Check sheet for the modelled part. Datum: model origin and axes. Units: mm. A direction names the side the tool comes from. Give positions to 0.01 mm unless a question says otherwise; leave off trailing zeros. Order: outer loops, then holes, each group sorted by start corner. A loop starts at its lowest first (then second) coordinate and runs counter-clockwise, first axis right, second up.
Autodesk Inventor part; units mm, degrees
ref_plane "YZ Plane" through (0, 0, 0) normal (1, 0, 0) x (0, 1, 0)
ref_plane "XZ Plane" through (0, 0, 0) normal (0, 1, 0) x (-1, 0, 0)
ref_plane "XY Plane" through (0, 0, 0) normal (0, 0, 1) x (1, 0, 0)
sketch "Sketch1" plane through (0, 0, 0) normal (1, 0, 0) x (0, 1, 0)
  line L0 (150, 0) -> (150, -150)
  line L1 (0, -150) -> (0, 0)
  line L2 (130, -42) -> (90, -42)
  line L3 (90, -42) -> (90, -138)
  line L4 (90, -138) -> (130, -138)
  line L5 (130, -138) -> (130, -42)
  line L6 (130, -42) -> (90, -138) construction
  line L7 (90, -42) -> (130, -138) construction
  line L8 (75, -77) -> (17, -77)
  line L9 (17, -77) -> (17, -138)
  line L10 (17, -138) -> (75, -138)
  line L11 (75, -138) -> (75, -77)
  line L12 (75, -77) -> (17, -138) construction
  line L13 (17, -77) -> (75, -138) construction
  line L14 (25, -30) -> (25, -60) construction
  line L15 (35, -30) -> (35, -60)
  line L16 (15, -60) -> (15, -30)
  arc A0 (35, -30) -> (15, -30) centre (25, -30) ccw
  arc A1 (15, -60) -> (35, -60) centre (25, -60) ccw
  line L17 (124, 0) -> (124, 10)
  line L18 (124, 10) -> (99, 10)
  line L19 (99, 10) -> (99, 0)
  line L20 (51, 0) -> (51, 10)
  line L21 (51, 10) -> (26, 10)
  line L22 (26, 10) -> (26, 0)
  line L23 (150, -75) -> (168, -75)
  line L24 (124, 0) -> (150, 0)
  line L25 (0, 0) -> (26, 0)
  line L26 (51, 0) -> (99, 0)
  line L27 (124, -150) -> (124, -160)
  line L28 (124, -160) -> (99, -160)
  line L29 (99, -160) -> (99, -150)
  line L30 (51, -150) -> (51, -160)
  line L31 (51, -160) -> (26, -160)
  line L32 (26, -160) -> (26, -150)
  line L33 (150, -150) -> (124, -150)
  line L34 (99, -150) -> (51, -150)
  line L35 (26, -150) -> (0, -150)
  point P0 (110, -90)
  point P1 (46, -107.5)
  point P2 (25, -45)
  dimension "d0" = 150
  dimension "d1" = 150
  dimension "d2" = 90
  dimension "d3" = 110
  dimension "d4" = 40
  dimension "d5" = 96
  dimension "d6" = 58
  dimension "d7" = 61
  dimension "d8" = 46
  dimension "d9" = 96
  dimension "d10" = 25
  dimension "d11" = 30
  dimension "d12" = 30
  dimension "d13" = 10
  dimension "d16" = 25
  dimension "d17" = 10
  dimension "d18" = 26
  dimension "d19" = 10
  dimension "d20" = 25
  dimension "d21" = 26
  dimension "d24" = 33
  dimension "d25" = 75
  dimension "d26" = 18
extrude "Extrusion1" add sketch "Sketch1" along normal blind 3
properties part number "front_part"
(1) Release check for a two-part mould opening along Z. For faces 1 (the face through (1, 25, -70)), 2 (the face through (0, 74, -74)) record: released by +Z, released by -Z, zero draft, split by the parting line, or undercut.
Response values:
face 1: undercut
face 2: zero draft
(2) Cross-section at C-C on x = 0.95. Count the separate pieces of the cut face and the enclosed holes in it, then the cut area to 3 significant figures.
Response values:
separate pieces: 1
enclosed holes: 3
area: 15,200 mm2
(3) Cross-section at A-A on y = 66. Enter the section's corners in (x, z), then the cut area to 3 significant figures.
Response values:
outline: (0, -150) - (3, -150) - (3, -138) - (0, -138) - close; (0, -77) - (3, -77) - (3, 0) - (0, 0) - close
area: 267 mm2
(4) Material ranges on L1, parallel to Y at x = 1.1, z = -132; L2, parallel to Z at x = 1.1, y = 21; L3, parallel to Z at x = 0.3, y = 118, recorded low to high.
Response values:
L1: y = 0 to 17, 75 to 90, 130 to 150
L2: z = -150 to -138, -77 to -69.17, -20.83 to 0
L3: z = -160 to -138, -42 to 10
(5) Set-up check for faces 3 (the face through (3, 74, -74)), 4 (the face through (1, 25, -20)): record each of +Z, -Z, +X, -X, +Y, -Y from which the full face is reachable in a straight line by a thin tool's end or side.
Response values:
face 3: +Z, -Z, +X, +Y, -Y
face 4: +X, -X
(6) Cross-section at B-B on z = -104.5. Enter the section's corners in (x, y), then the cut area to 3 significant figures.
Response values:
outline: (0, 0) - (3, 0) - (3, 17) - (0, 17) - close; (0, 75) - (3, 75) - (3, 90) - (0, 90) - close; (0, 130) - (3, 130) - (3, 150) - (0, 150) - close
area: 156 mm2
(7) Gauge pin test, flat ends, axial feed: pin 1 Ø0.9 at (x, z) = (2, -155) entering from +Y; pin 2 Ø1.5 at (x, z) = (1, 7) entering from -Y; pin 3 Ø5 at (y, z) = (22.5, -80.5) entering from -X. Record the tip position at first contact, or that the pin passes through.
Response values:
pin 1: stops at y = 124
pin 2: stops at y = 26
pin 3: passes through
(8) Cross-section at D-D on y = 116. Enter the section's corners in (x, z).
Response values:
outline: (0, -160) - (3, -160) - (3, -138) - (0, -138) - close; (0, -42) - (3, -42) - (3, 10) - (0, 10) - close
